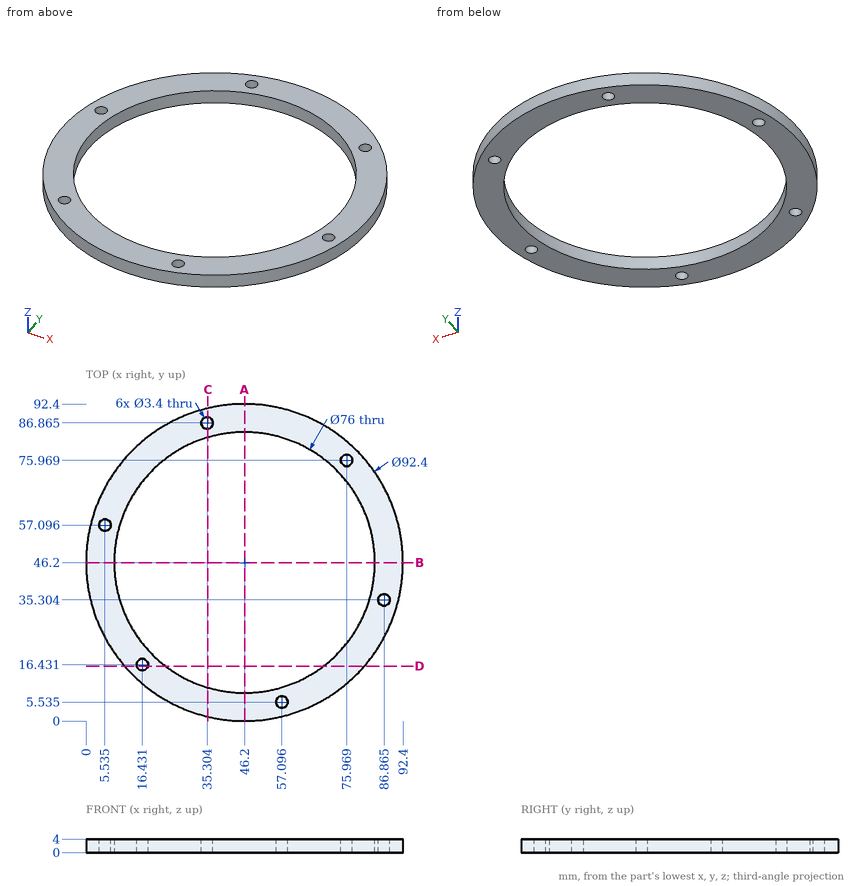
Can you work these out from the drawing? Everything is in mm from the part's minimum corner. Round coordinates to 2 decimals unless told otherwise and drop trailing zeros. Order: outer loops, then holes, each group sorted by start corner. A loop starts at its lowest first (then second) coordinate and runs counter-clockwise, first axis right, second up.
(1) If I drill on L1, parallel to Y at x = 16.5, z = 1.6 (1 decimal); L2, parallel to Y at x = 57.5, z = 2.4 (1 decimal); L3, parallel to X at y = 76.5, z = 1.55 (1 decimal), over which ranges is the centre line in solid material (lowest first)?
Results are:
L1: y = 10.8 to 14.7, 18.1 to 22.5, 69.9 to 81.6
L2: y = 1.4 to 3.9, 7.2 to 9.9, 82.5 to 91
L3: x = 11.3 to 23.3, 69.1 to 74.4, 77.6 to 81.1
(2) If we section it at A-A (x = 46.2): Please give me the cut outline in (y, z).
Results are:
outline: (0, 0) - (8.2, 0) - (8.2, 4) - (0, 4) - close; (84.2, 0) - (92.4, 0) - (92.4, 4) - (84.2, 4) - close
(3) If we section it at C-C (x = 35.5): Please give me the cut outline in (y, z) (1 decimal).
Results are:
outline: (1.3, 0) - (9.7, 0) - (9.7, 4) - (1.3, 4) - close; (82.7, 0) - (85.2, 0) - (85.2, 4) - (82.7, 4) - close; (88.6, 0) - (91.1, 0) - (91.1, 4) - (88.6, 4) - close
(4) If we section it at D-D (y = 16): Please give me the cut outline in (x, z) (1 decimal).
Results are:
outline: (11.2, 0) - (14.8, 0) - (14.8, 4) - (11.2, 4) - close; (18.1, 0) - (23.1, 0) - (23.1, 4) - (18.1, 4) - close; (69.3, 0) - (81.2, 0) - (81.2, 4) - (69.3, 4) - close
(5) I'm going to push flat-ended pins straight in: pin 1 (1.5 mm diameter, centred on y = 64, z = 1, fed in from +X); pin 2 (1.5 mm diameter, centred on y = 27.5, z = 0.5, fed in from -X); pin 3 (3 mm diameter, centred on x = 86.87, y = 35.3, fed in from -Z); pin 4 (1 mm diameter, centred on y = 19, z = 1.5, fed in from -X). Where does each tip first touch, or does it pass through?
Results are:
pin 1: stops at x = 89.14
pin 2: stops at x = 3.63
pin 3: passes through
pin 4: stops at x = 8.5
